from build123d import *

# Parameters (mm, degrees)
F0_W     = 1066.8
F0_H     = 88.9
F1_DEPTH = 19.05
F2_W     = 4.7625
F2_H     = 13.97
F3_DEPTH = 1066.801
F5_DEPTH = 19.051


with BuildPart() as f1:
    # F0 (on Front) → F1 (new body)
    with BuildSketch(Plane.XZ):
        with Locations((0, 44.45)):
            Rectangle(F0_W, F0_H)
    extrude(amount=F1_DEPTH)

    # F2 (on face) → F3 (cut, through all)
    with BuildSketch(Plane.YZ.offset(533.4)):
        with Locations((-2.38125, 6.985)):
            Rectangle(F2_W, F2_H)
    extrude(amount=-F3_DEPTH, mode=Mode.SUBTRACT)

    # F4 (on face) → F5 (cut, through all)
    with BuildSketch(Plane.XZ.offset(19.05)):
        Polygon((-444.5, 0), (-533.4, 88.9), (-533.4, 0), align=None)
        Polygon((444.5, 0), (533.4, 0), (533.4, 88.9), align=None)
    extrude(amount=-F5_DEPTH, mode=Mode.SUBTRACT)


solid = f1.part
Verification items for the finished model (mm, model axes). Give positions to 0.01 mm unless a question says otherwise; leave off trailing zeros. Write each loop counter-clockwise with the first axis right and the second up, starting at its lowest first coordinate (ties: lowest second). Pieces come first, ordered by that corner, then holes. Notation, with made-up numbers: M 76.25,58.25 L 102.25,58.25 A14 ccw 102.25,71.25 Z; hole C 74.25,36 d6. An arc over 180 degrees is marked long. Use CSV: the item, a comma, the result in double quotes.
1) Go/stop test with flat-tipped pins: pin 1 Ø6 at (y, z) = (-11, 36) entering from -X; pin 2 Ø15.5 at (x, z) = (-92.5, 4.5) entering from +Y; pin 3 Ø2 at (y, z) = (-16, 72) entering from +X. Record where each tip stops, or that it passes through.
Final values:
pin 1,"x = -483.5"
pin 2,"y = -4.76"
pin 3,"x = 517.5"
2) Cross-section at C-C (y = -15.75). Enter the section's corners in (x, z), plus the area to 3 significant figures.
Final values:
outline,"M -533.4,88.9 L -444.5,0 L 444.5,0 L 533.4,88.9 Z"
area,"86,900 mm²"
3) Cross-section at B-B (z = 24). Enter the section's corners in (x, y).
Final values:
outline,"M -468.5,-19.05 L 468.5,-19.05 L 468.5,0 L -468.5,0 Z"
4) Material ranges on line 1 along Y through (x, z) = (215, 7.5); line 2 along Z through (x, y) = (214.5, -1.75); line 3 along X through (y, z) = (-15, 54.5), recorded low to high.
Final values:
line 1,"-19.05 to -4.76"
line 2,"13.97 to 88.9"
line 3,"-499 to 499"
5) Cross-section at A-A (x = -123). Enter the section's corners in (y, z), plus the area to 3 significant figures.
Final values:
outline,"M -19.05,0 L -4.76,0 L -4.76,13.97 L 0,13.97 L 0,88.9 L -19.05,88.9 Z"
area,"1,630 mm²"
